Autodesk Inventor part; units mm, degrees
ref_plane "YZ Plane" through (0, 0, 0) normal (1, 0, 0) x (0, 1, 0)
ref_plane "XZ Plane" through (0, 0, 0) normal (0, 1, 0) x (-1, 0, 0)
ref_plane "XY Plane" through (0, 0, 0) normal (0, 0, 1) x (1, 0, 0)
sketch "Эскиз1" plane through (0, 0, 0) normal (0, 0, 1) x (1, 0, 0)
  circle A0 centre (0, 0) radius 33
  circle A1 centre (0, 0) radius 32
  arc A2 (-5.4738, 32.5429) -> (-3.8704, 34.0101) centre (-5.8055, 34.5152) ccw
  arc A3 (3.8704, 34.0101) -> (-3.8704, 34.0101) centre (0, 33) ccw
  arc A4 (3.8704, 34.0101) -> (5.4738, 32.5429) centre (5.8055, 34.5152) ccw
  line L0 (-19, -25.7488) -> (19, -25.7488) construction
  line L1 (-19, -25.7488) -> (-19.8409, -26.3693)
  line L2 (19, -25.7488) -> (19.5938, -26.5534)
  arc A5 (-5.3079, 31.5567) -> (-2.9028, 33.7576) centre (-5.8055, 34.5152) ccw
  arc A6 (2.9028, 33.7576) -> (-2.9028, 33.7576) centre (0, 33) ccw
  arc A7 (2.9028, 33.7576) -> (5.3079, 31.5567) centre (5.8055, 34.5152) ccw
  point P0 (5.3079, 31.5567)
  point P1 (-5.3079, 31.5567)
  dimension "d0" = 66
  dimension "d1" = 64
  dimension "d2" = 4
  dimension "d4" = 2
  dimension "d5" = 38
extrude "Выдавливание1" add sketch "Эскиз1" along normal mid plane 1 contours A0 L2 A1 A7 | A0 A7 A6 A5 A2 A3 A4 | A0 A5 A1 L1
properties part number "69. Пружина синхронизатора"
Could you check a few things on this model? Use its own coordinates, in mm. A direction names the side the tool comes from. Round coordinates to 2 decimals unless told otherwise and drop trailing zeros. Write each loop counter-clockwise with the first axis right and the second up, starting at its lowest first coordinate (ties: lowest second). Pieces come first, ordered by that corner, then holes. Notation, with made-up numbers: M 62.25,-29 L 89.25,-29 A25 ccw 89.25,-7 Z; hole C -20,-21.75 d7. An arc over 180 degrees is marked long. Answer in a Markdown table with one row per item. Add a question column.
Q1. If I drill on line 1 (X direction, y = -0.5, z = 0.35); line 2 (X direction, y = 27, z = 0.3); line 3 (Y direction, x = 25, z = -0.2), over which ranges is the centre line in solid material (lowest first)? Write a range as from..to.
Q2. On a 3-axis mill with a long thin cutter (end or side, diameter ignored), from which of +Z, -Z, +X, -X, +Y, -Y can I reach the whole of each face in a straight line? I mean faces 1 (the cylindrical face through (3.798, 32.286, -0.007)), 2 (the flat face through (-7.5, 31.3, -0.5)). Say none if no direction works.
Q3. Imagine slicing it at C-C (z = 0.2). Please give me the cut outline in (x, y), then the cut area to 3 significant figures.
Q4. Imagine slicing it at B-B (x = -24.5). Please give me the cut outline in (y, z), then the cut area to 4 significant figures.
Q5. If we mould it in two halves opening along Y, with no side actions, what happens to faces 3 (the cylindrical face through (0, 37, 0)), 4 (the cylindrical face through (0, 36, 0)), 5 (the cylindrical face through (30.998, 7.945, -0.007)), 6 (the cylindrical face through (-31.24, 6.93, -0.01))? For each: +Y half, -Y half, draft (parallel to the pull), parting line (faces both ways), or undercut.
Q6. Imagine slicing it at D-D (x = -13). Please give me the cut outline in (y, z).
Q7. Imagine slicing it at A-A (y = 28.5). Please give me the cut outline in (x, z).
Values:
| question | item | result |
|---|---|---|
| 1 | line 1 | -33..-32, 32..33 |
| 1 | line 2 | -18.97..-17.18, 17.18..18.97 |
| 1 | line 3 | -21.54..-19.97, 19.97..21.54 |
| 2 | face 1 | +Z, -Z, -Y |
| 2 | face 2 | -Z, +X, -X, +Y, -Y |
| 3 | outline | M -19.84,-26.37 L -19,-25.75 A32 cw -5.31,31.56 A3 ccw -2.9,33.76 A3 cw 2.9,33.76 A3 ccw 5.31,31.56 A32 cw 19,-25.75 L 19.59,-26.55 A33 ccw 5.47,32.54 A2 cw 3.87,34.01 A4 ccw -3.87,34.01 A2 cw -5.47,32.54 A33 ccw Z |
| 3 | area | 167 mm^2 |
| 4 | outline | M -22.11,-0.5 L -20.59,-0.5 L -20.59,0.5 L -22.11,0.5 Z; M 20.59,-0.5 L 22.11,-0.5 L 22.11,0.5 L 20.59,0.5 Z |
| 4 | area | 3.045 mm^2 |
| 5 | face 3 | +Y half |
| 5 | face 4 | -Y half |
| 5 | face 5 | undercut |
| 5 | face 6 | undercut |
| 6 | outline | M 29.24,-0.5 L 30.33,-0.5 L 30.33,0.5 L 29.24,0.5 Z |
| 7 | outline | M -16.64,-0.5 L -14.55,-0.5 L -14.55,0.5 L -16.64,0.5 Z; M 14.55,-0.5 L 16.64,-0.5 L 16.64,0.5 L 14.55,0.5 Z |
